Input: part model. Units: mm. Frame: model coordinates. Face numbers are marked on the shaded views. Coordinates: 2 decimals unless noted, no trailing zeros. Order: outer loops, then holes, each group sorted by start corner. A loop starts at its lowest first (then second) coordinate and runs counter-clockwise, first axis right, second up. Notation, with made-up numbers: (44, 66) - (52, 66) arc R10 ccw to (52, 80) - close; hole circle Ø7 at (46.5, 31). An arc over 180 degrees is marked (long way). Answer as CSV lines item,"result". Start each with the question number.
Item 1: Section D-D (y = 27). Output: boundary loops of the cut face in (x, z), and give its area (3 significant figures).
Item 2: Draft query along Y for the marked faces 1 and 2. Return one class per face: +Y half, -Y half, draft (parallel to the pull), parting line (faces both ways), or undercut.
Item 3: First-contact query: pin 1 (4 mm diameter, centred on x = 36, z = 120, fed in from -Y); pin 2 (8 mm diameter, centred on y = 61, z = 82, fed in from +X); pin 3 (12 mm diameter, centred on y = -69, z = 223.5, fed in from +X). Flat tips, straight axial feed; report the tip coordinate or a pass-through.
Item 4: Material intervals for line 1 along Z through (x, y) = (0, -87.55); line 2 along Y through (x, z) = (0, 76); line 3 along Y through (x, z) = (-44.5, 238), sorted ascending.
Item 5: Section A-A (y = 0). Output: boundary loops of the cut face in (x, z), and give its area (3 significant figures).
Item 6: Section B-B (z = 149.5). Output: boundary loops of the cut face in (x, y), and give its area (3 significant figures).
Item 7: Section C-C (x = 26.5). Output: boundary loops of the cut face in (y, z).
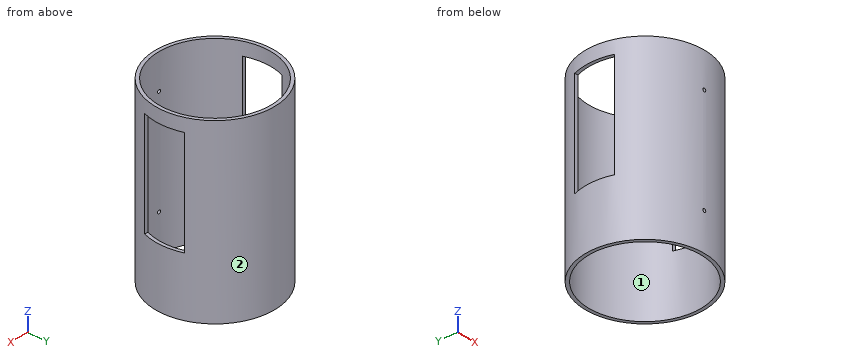
from build123d import *

# Parameters (mm, degrees)
SKETCH1_R               = 90
SKETCH1_R_2             = 85
BOSS_EXTRUDE1_DEPTH     = 270
SKETCH2_W               = 160
SKETCH2_H               = 60
CUT_EXTRUDE1_DEPTH      = 81
CUT_EXTRUDE1_DEPTH_BACK = 101
SKETCH3_R               = 2.5
CUT_EXTRUDE2_DEPTH      = 200


with BuildPart() as part:
    # Sketch1 → Boss-Extrude1 (new body)
    with BuildSketch(Plane.XY):
        Circle(SKETCH1_R)
        Circle(SKETCH1_R_2, mode=Mode.SUBTRACT)
    extrude(amount=BOSS_EXTRUDE1_DEPTH)

    # Sketch2 → Cut-Extrude1 (cut, two sides)
    with BuildSketch(Plane(origin=(10, 0, 0), x_dir=(0, 0, -1), z_dir=(1, 0, 0))) as cut_extrude1_sk:
        with Locations((-170, 0)):
            Rectangle(SKETCH2_W, SKETCH2_H)
    extrude(amount=CUT_EXTRUDE1_DEPTH, mode=Mode.SUBTRACT)
    extrude(cut_extrude1_sk.sketch, amount=-CUT_EXTRUDE1_DEPTH_BACK, mode=Mode.SUBTRACT)

    # Sketch3 → Cut-Extrude2 (cut)
    with BuildSketch(Plane(origin=(0, 10, 0), x_dir=(1, 0, 0), z_dir=(0, 1, 0))):
        with Locations((0, -216.93551415)):
            Circle(SKETCH3_R)
        with Locations((0, -56.93551415)):
            Circle(SKETCH3_R)
    extrude(amount=-CUT_EXTRUDE2_DEPTH, mode=Mode.SUBTRACT)


solid = part.part
Determined:
1,outline,"(-85.85, 0) - (-80.6, 0) - (-80.6, 90) - (-85.85, 90) - close; (-85.85, 250) - (-80.6, 250) - (-80.6, 270) - (-85.85, 270) - close; (80.6, 0) - (85.85, 0) - (85.85, 90) - (80.6, 90) - close; (80.6, 250) - (85.85, 250) - (85.85, 270) - (80.6, 270) - close"
1,area,"1,160 mm^2"
2,face 1,"undercut"
2,face 2,"parting line"
3,pin 1,"stops at y = -83.33"
3,pin 2,"stops at x = 69.65"
3,pin 3,"stops at x = 64.27"
4,line 1,"z = 0 to 54.44, 59.44 to 214.44, 219.44 to 270"
4,line 2,"y = -90 to -85, 85 to 90"
4,line 3,"y = -78.23 to -72.42, 72.42 to 78.23"
5,outline,"(-90, 0) - (-85, 0) - (-85, 90) - (-90, 90) - close; (-90, 250) - (-85, 250) - (-85, 270) - (-90, 270) - close; (85, 0) - (90, 0) - (90, 90) - (85, 90) - close; (85, 250) - (90, 250) - (90, 270) - (85, 270) - close"
5,area,"1,100 mm^2"
6,outline,"(-84.85, -30) arc R90 ccw to (84.85, -30) - (79.53, -30) arc R85 cw to (-79.53, -30) - close; (-84.85, 30) - (-79.53, 30) arc R85 cw to (79.53, 30) - (84.85, 30) arc R90 ccw to start"
6,area,"2,140 mm^2"
7,outline,"(-86.01, 0) - (-80.76, 0) - (-80.76, 270) - (-86.01, 270) - close; (80.76, 0) - (86.01, 0) - (86.01, 270) - (80.76, 270) - close"
